```python
from build123d import *

# Parameters (mm, degrees)
SKETCH1_R           = 5
SKETCH1_R_2         = 3.5
BOSS_EXTRUDE1_DEPTH = 10.5
SKETCH4_R           = 11
SKETCH4_R_2         = 5
BOSS_EXTRUDE2_DEPTH = 3.5
SKETCH5_R           = 1.25
CUT_EXTRUDE2_DEPTH  = 19.768324379
CHAMFER1_SIZE       = 0.2


with BuildPart() as part:
    # Sketch1 → Boss-Extrude1 (new body)
    with BuildSketch(Plane(origin=(0, 0, 0), x_dir=(1, 0, 0), z_dir=(0, 1, 0))):
        with Locations(Location((0, 0, 0), (0, 0, 90))):
            Circle(SKETCH1_R)
        with Locations(Location((0, 0, 0), (0, 0, 90))):
            Circle(SKETCH1_R_2, mode=Mode.SUBTRACT)
    extrude(amount=BOSS_EXTRUDE1_DEPTH)

    # Sketch4 → Boss-Extrude2 (add)
    with BuildSketch(Plane(origin=(0, 2, 0), x_dir=(1, 0, 0), z_dir=(0, 1, 0))):
        with Locations(Location((0, 0, 0), (0, 0, 270))):
            Circle(SKETCH4_R)
        with Locations(Location((0, 0, 0), (0, 0, 90))):
            Circle(SKETCH4_R_2, mode=Mode.SUBTRACT)
    extrude(amount=BOSS_EXTRUDE2_DEPTH)

    # Sketch5 → Cut-Extrude2 (cut, through all)
    with BuildSketch(Plane(origin=(0, 0, 0), x_dir=(1, 0, 0), z_dir=(0, 1, 0))):
        with Locations(Location((-6, 6, 0), (0, 0, 90))):
            Circle(SKETCH5_R)
        with Locations(Location((6, 6, 0), (0, 0, 90))):
            Circle(SKETCH5_R)
        with Locations(Location((6, -6, 0), (0, 0, 90))):
            Circle(SKETCH5_R)
        with Locations(Location((-6, -6, 0), (0, 0, 90))):
            Circle(SKETCH5_R)
    extrude(amount=CUT_EXTRUDE2_DEPTH, mode=Mode.SUBTRACT)

    # Chamfer1
    chamfer1_edges = [part.edges().sort_by_distance(p)[0] for p in [
        (0, 5.5, -11),
        (0, 2, -11),
        (-6, 5.5, -4.75),
        (-6, 2, -4.75),
        (0, 0, 5),
        (6, 5.5, -4.75),
        (6, 2, -4.75),
        (6, 5.5, 7.25),
        (6, 2, 7.25),
        (-6, 5.5, 7.25),
        (-6, 2, 7.25),
        (0, 10.5, 5),
        (0, 0, 3.5),
        (0, 10.5, 3.5),
    ]]
    chamfer(chamfer1_edges, length=CHAMFER1_SIZE)


solid = part.part
```
CAD build for the part. Positions are in the model's coordinates, mm. A direction names the side the tool comes from. Give positions to 0.01 mm unless a question says otherwise; leave off trailing zeros. Order: outer loops, then holes, each group sorted by start corner. A loop starts at its lowest first (then second) coordinate and runs counter-clockwise, first axis right, second up.
(1) Drill centre lines: L1, parallel to Z at x = 5.75, y = 3.75; L2, parallel to X at y = 3.8, z = -6; L3, parallel to Y at x = -6.75, z = 3.25. Where is each one in solid material? Low to high.
(2) Mould opens along Z. For faces 1 (the cylindrical face through (4.88, 1.09, 1.08)), 2 (the cylindrical face through (7.22, 3.73, -5.73)), 3 (the flat face through (4, 10.5, -1)) say: released by +Z, released by -Z, zero draft, split by the parting line, or undercut.
(3) Saw through at B-B, the plane z = 0. Give the cut face in (x, y).
(4) Flat gauge pins, fed straight in: pin 1 (3 mm diameter, centred on x = -6, z = 6, fed in from +Y); pin 2 (4 mm diameter, centred on x = 6, z = -6, fed in from -Y); pin 3 (2 mm diameter, centred on y = 7.5, z = 0, fed in from -X). Where does each tip first touch, or does it go through?
(5) Saw through at D-D, the plane x = -6.5. State how many separate pieces and enclosed holes the cut face has, then the cut area to 3 significant figures.
(6) Tool access for faces 4 (the flat face through (-2, 5.5, 5)), 5 (the cylindrical face through (-4.78, 3.73, 6.27)): list every direction of +Z, -Z, +X, -X, +Y, -Y with a clear straight run to the whole face (end or side of a thin tool).
(7) Saw through at C-C, the plane y = 8.5. Give the cut face in (x, z).
(8) Saw through at A-A, the plane x = 0. Give the cut face in (y, z), then the cut area to 3 significant figures.
Results found:
1. L1: z = -9.38 to -7.22, -4.78 to 4.78, 7.22 to 9.38
1. L2: x = -9.22 to -7.25, -4.75 to 4.75, 7.25 to 9.22
1. L3: y = 2 to 5.5
2. face 1: split by the parting line
2. face 2: undercut
2. face 3: zero draft
3. outline: (-11, 2.2) - (-10.8, 2) - (-5, 2) - (-5, 0.2) - (-4.8, 0) - (-3.7, 0) - (-3.5, 0.2) - (-3.5, 10.3) - (-3.7, 10.5) - (-4.8, 10.5) - (-5, 10.3) - (-5, 5.5) - (-10.8, 5.5) - (-11, 5.3) - close; (3.5, 0.2) - (3.7, 0) - (4.8, 0) - (5, 0.2) - (5, 2) - (10.8, 2) - (11, 2.2) - (11, 5.3) - (10.8, 5.5) - (5, 5.5) - (5, 10.3) - (4.8, 10.5) - (3.7, 10.5) - (3.5, 10.3) - close
4. pin 1: stops at y = 5.5
4. pin 2: stops at y = 2
4. pin 3: stops at x = -5
5. separate pieces: 3
5. enclosed holes: 0
5. area: 45.8 mm2
6. face 4: +Y
6. face 5: +Y, -Y
7. outline: circle Ø10 at (0, 0); hole circle Ø7 at (0, 0)
8. outline: (0, -4.8) - (0.2, -5) - (2, -5) - (2, -10.8) - (2.2, -11) - (5.3, -11) - (5.5, -10.8) - (5.5, -5) - (10.3, -5) - (10.5, -4.8) - (10.5, -3.7) - (10.3, -3.5) - (0.2, -3.5) - (0, -3.7) - close; (0, 3.7) - (0.2, 3.5) - (10.3, 3.5) - (10.5, 3.7) - (10.5, 4.8) - (10.3, 5) - (5.5, 5) - (5.5, 10.8) - (5.3, 11) - (2.2, 11) - (2, 10.8) - (2, 5) - (0.2, 5) - (0, 4.8) - close
8. area: 73.3 mm2
